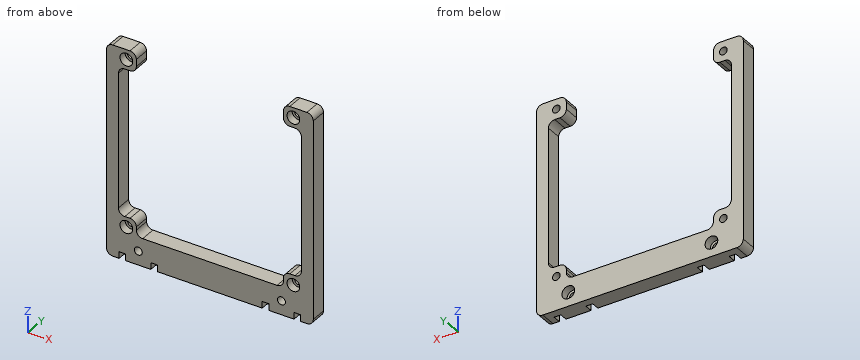
from build123d import *

# Parameters (mm, degrees)
SKETCH1_W           = 130
SKETCH1_H           = 132.5
BOSS_EXTRUDE1_DEPTH = 10
SKETCH2_R           = 2.4
CUT_EXTRUDE1_DEPTH  = 94.349143006
SKETCH3_W           = 115
SKETCH3_H           = 92.5
CUT_EXTRUDE2_DEPTH  = 94.349143006
SKETCH5_W           = 92.5
SKETCH5_H           = 115
CUT_EXTRUDE3_DEPTH  = 94.349143006
FILLET1_R           = 4
SKETCH6_R           = 2.5
CUT_EXTRUDE4_DEPTH  = 10
SKETCH7_R           = 4
CUT_EXTRUDE5_DEPTH  = 5
SKETCH8_W           = 4.2
SKETCH8_H           = 4.2
CUT_EXTRUDE6_DEPTH  = 5
SKETCH9_R           = 4
CUT_EXTRUDE7_DEPTH  = 5


with BuildPart() as part:
    # Sketch1 → Boss-Extrude1 (new body)
    with BuildSketch(Plane(origin=(0, 0, 0), x_dir=(1, 0, 0), z_dir=(0, 1, 0))):
        Rectangle(SKETCH1_W, SKETCH1_H)
    extrude(amount=BOSS_EXTRUDE1_DEPTH)

    # Sketch2 → Cut-Extrude1 (cut, through all)
    with BuildSketch(Plane(origin=(0, 10, 0), x_dir=(1, 0, 0), z_dir=(0, 1, 0))):
        with Locations(Location((-52.5, -60, 0), (0, 0, 270))):
            Circle(SKETCH2_R)
        with Locations(Location((52.5, -60, 0), (0, 0, 270))):
            Circle(SKETCH2_R)
        with Locations(Location((52.5, 45, 0), (0, 0, 270))):
            Circle(SKETCH2_R)
        with Locations(Location((-52.5, 45, 0), (0, 0, 270))):
            Circle(SKETCH2_R)
    extrude(amount=-CUT_EXTRUDE1_DEPTH, mode=Mode.SUBTRACT)

    # Sketch3 → Cut-Extrude2 (cut, through all)
    with BuildSketch(Plane(origin=(0, 10, 0), x_dir=(1, 0, 0), z_dir=(0, 1, 0))):
        with Locations((0, -7.5)):
            Rectangle(SKETCH3_W, SKETCH3_H)
    extrude(amount=-CUT_EXTRUDE2_DEPTH, mode=Mode.SUBTRACT)

    # Sketch5 → Cut-Extrude3 (cut, through all)
    with BuildSketch(Plane(origin=(0, 10, 0), x_dir=(1, 0, 0), z_dir=(0, 1, 0))):
        with Locations((0, -8.75)):
            Rectangle(SKETCH5_W, SKETCH5_H)
    extrude(amount=-CUT_EXTRUDE3_DEPTH, mode=Mode.SUBTRACT)

    # Fillet1
    fillet1_edges = [part.edges().sort_by_distance(p)[0] for p in [
        (-57.5, 5, 53.75),
        (-57.5, 5, -38.75),
        (57.5, 5, -38.75),
        (57.5, 5, 53.75),
        (46.25, 5, 53.75),
        (-46.25, 5, 53.75),
        (-46.25, 5, -38.75),
        (-46.25, 5, 66.25),
        (46.25, 5, -38.75),
        (46.25, 5, -48.75),
        (-46.25, 5, -48.75),
        (46.25, 5, 66.25),
        (65, 5, 66.25),
        (-65, 5, 66.25),
        (-65, 5, -66.25),
        (65, 5, -66.25),
    ]]
    fillet(fillet1_edges, radius=FILLET1_R)

    # Sketch6 → Cut-Extrude4 (cut)
    with BuildSketch(Plane(origin=(0, 10, 0), x_dir=(1, 0, 0), z_dir=(0, 1, 0))):
        with Locations(Location((-45, 57.5, 0), (0, 0, 270))):
            Circle(SKETCH6_R)
        with Locations(Location((45, 57.5, 0), (0, 0, 270))):
            Circle(SKETCH6_R)
    extrude(amount=-CUT_EXTRUDE4_DEPTH, mode=Mode.SUBTRACT)

    # Sketch7 → Cut-Extrude5 (cut)
    with BuildSketch(Plane(origin=(0, 10, 0), x_dir=(1, 0, 0), z_dir=(0, 1, 0))):
        with Locations(Location((-45, 57.5, 0), (0, 0, 270))):
            Circle(SKETCH7_R)
        with Locations(Location((45, 57.5, 0), (0, 0, 270))):
            Circle(SKETCH7_R)
    extrude(amount=-CUT_EXTRUDE5_DEPTH, mode=Mode.SUBTRACT)

    # Sketch8 → Cut-Extrude6 (cut)
    with BuildSketch(Plane(origin=(0, 0, 0), x_dir=(1, 0, 0), z_dir=(0, 1, 0))):
        with Locations((-55, 64.15)):
            Rectangle(SKETCH8_W, SKETCH8_H)
        with Locations((-35, 64.15)):
            Rectangle(SKETCH8_W, SKETCH8_H)
        with Locations((35, 64.15)):
            Rectangle(SKETCH8_W, SKETCH8_H)
        with Locations((55, 64.15)):
            Rectangle(SKETCH8_W, SKETCH8_H)
    extrude(amount=CUT_EXTRUDE6_DEPTH, mode=Mode.SUBTRACT)

    # Sketch9 → Cut-Extrude7 (cut)
    with BuildSketch(Plane.XZ):
        with Locations(Location((-52.5, 60, 0), (0, 0, 270))):
            Circle(SKETCH9_R)
        with Locations(Location((52.5, 60, 0), (0, 0, 270))):
            Circle(SKETCH9_R)
        with Locations(Location((-52.5, -45, 0), (0, 0, 270))):
            Circle(SKETCH9_R)
        with Locations(Location((52.5, -45, 0), (0, 0, 270))):
            Circle(SKETCH9_R)
    extrude(amount=-CUT_EXTRUDE7_DEPTH, mode=Mode.SUBTRACT)


solid = part.part
Verification items for the finished model (mm, model axes). Round coordinates to 2 decimals unless told otherwise and drop trailing zeros. Write each loop counter-clockwise with the first axis right and the second up, starting at its lowest first coordinate (ties: lowest second). Pieces come first, ordered by that corner, then holes.
(1) Section check D-D (x = 39). Enter the section's corners in (y, z).
Returned:
outline: (0, -66.25) - (10, -66.25) - (10, -48.75) - (0, -48.75) - close
(2) Section check B-B (z = -57.5). Enter the section's corners in (x, y).
Returned:
outline: (-65, 0) - (-47.5, 0) - (-47.5, 5) - (-49, 5) - (-49, 10) - (-65, 10) - close; (-42.5, 0) - (42.5, 0) - (42.5, 5) - (41, 5) - (41, 10) - (-41, 10) - (-41, 5) - (-42.5, 5) - close; (47.5, 0) - (65, 0) - (65, 10) - (49, 10) - (49, 5) - (47.5, 5) - close
(3) Material ranges on line 1 (X direction, y = 3.8, z = -45); line 2 (X direction, y = 8.3, z = -57.5); line 3 (X direction, y = 6.1, z = 60), recorded low to high.
Returned:
line 1: x = -65 to -56.5, -48.5 to -46.24, 46.24 to 48.5, 56.5 to 65
line 2: x = -65 to -49, -41 to 41, 49 to 65
line 3: x = -65 to -54.9, -50.1 to -46.25, 46.25 to 50.1, 54.9 to 65
(4) Section check C-C (z = 60). Enter the section's corners in (x, y).
Returned:
outline: (-65, 0) - (-56.5, 0) - (-56.5, 5) - (-54.9, 5) - (-54.9, 10) - (-65, 10) - close; (-50.1, 5) - (-48.5, 5) - (-48.5, 0) - (-46.25, 0) - (-46.25, 10) - (-50.1, 10) - close; (46.25, 0) - (48.5, 0) - (48.5, 5) - (50.1, 5) - (50.1, 10) - (46.25, 10) - close; (54.9, 5) - (56.5, 5) - (56.5, 0) - (65, 0) - (65, 10) - (54.9, 10) - close
(5) Section check A-A (z = -5.5). Enter the section's corners in (x, y).
Returned:
outline: (-65, 0) - (-57.5, 0) - (-57.5, 10) - (-65, 10) - close; (57.5, 0) - (65, 0) - (65, 10) - (57.5, 10) - close
(6) Depth check by flat-ended pin: pin 1 Ø5.5 at (x, z) = (52.5, -45) entering from -Y; pin 2 Ø1.3 at (x, y) = (-55, 2) entering from -Z; pin 3 Ø3 at (x, y) = (15.5, 3) entering from +Z. Enter the tip coordinate at first touch or a pass-through.
Returned:
pin 1: stops at y = 5
pin 2: stops at z = -62.05
pin 3: stops at z = -48.75
